Source: CAD feature listing. Evaluate the final solid. Frame: model axes, mm. Face numbers are marked on the shaded views. Give positions to 0.01 mm unless a question says otherwise; leave off trailing zeros. Loops run counter-clockwise (first coordinate to the right, second up) from the corner with the lowest first, then second, coordinate; pieces in that order, holes last. Notation, with made-up numbers: M 36,-1 L 89,-1 A30 cw 89,29 Z; hole C 59.25,-19 d7. An arc over 180 degrees is marked long. Answer in a Markdown table with one row per item.
```python
from build123d import *

# Parameters (mm, degrees)
SKETCH1_W           = 12
SKETCH1_H           = 30
BOSS_EXTRUDE1_DEPTH = 5
SKETCH2_R           = 2.25
CUT_EXTRUDE1_DEPTH  = 153.676695316
CHAMFER1_SIZE       = 2


with BuildPart() as part:
    # Sketch1 → Boss-Extrude1 (new body)
    with BuildSketch(Plane.XY):
        with Locations((127.56172091, 58.8)):
            Rectangle(SKETCH1_W, SKETCH1_H)
    extrude(amount=BOSS_EXTRUDE1_DEPTH)

    # Sketch2 → Cut-Extrude1 (cut, through all)
    with BuildSketch(Plane.XY.offset(5)):
        with Locations((127.56172091, 67.8)):
            Circle(SKETCH2_R)
        with Locations((127.56172091, 49.8)):
            Circle(SKETCH2_R)
    extrude(amount=-CUT_EXTRUDE1_DEPTH, mode=Mode.SUBTRACT)

    # Chamfer1
    # the kernel refuses this chamfer: 2 mm, written as the material it takes off along each edge
    with BuildSketch(Plane(origin=(133.56172091, 38.656634024, 5), x_dir=(0.027495876610582174, 0, -0.9996219169112968), z_dir=(0, 1, 0)), Plane(origin=(121.56172091, 78.943365976, 5), x_dir=(-0.02749587661058908, 0, -0.9996219169112968), z_dir=(0, -1, 0))) as chamfer1_piece_1:
        Polygon((CHAMFER1_SIZE * 0.999621916911, CHAMFER1_SIZE * 0.0274958766106), (-CHAMFER1_SIZE * 0.0274958766106, CHAMFER1_SIZE * 0.999621916911), (0, 0), align=None)
    extrude(amount=40.286731952, mode=Mode.SUBTRACT)
    with BuildSketch(Plane(origin=(127.56172091, 67.8, 5), x_dir=(1, 0, 0), z_dir=(0, -1, 0))) as chamfer1_piece_2:
        Polygon((2.25 + CHAMFER1_SIZE, 0), (2.25, -CHAMFER1_SIZE), (2.25, 0), align=None)
    revolve(axis=Axis((127.56172091, 67.8, 5), (0, 0, 1)), mode=Mode.SUBTRACT)
    with BuildSketch(Plane(origin=(138.705086886, 73.8, 5), x_dir=(0, 0.02749587661058908, -0.9996219169112968), z_dir=(-1, 0, 0))) as chamfer1_piece_3:
        Polygon((CHAMFER1_SIZE * 0.999621916911, CHAMFER1_SIZE * 0.0274958766106), (-CHAMFER1_SIZE * 0.0274958766106, CHAMFER1_SIZE * 0.999621916911), (0, 0), align=None)
    extrude(amount=22.286731952, mode=Mode.SUBTRACT)
    with BuildSketch(Plane(origin=(127.56172091, 49.8, 5), x_dir=(1, 0, 0), z_dir=(0, -1, 0))) as chamfer1_piece_4:
        Polygon((2.25 + CHAMFER1_SIZE, 0), (2.25, -CHAMFER1_SIZE), (2.25, 0), align=None)
    revolve(axis=Axis((127.56172091, 49.8, 5), (0, 0, 1)), mode=Mode.SUBTRACT)
    with BuildSketch(Plane(origin=(116.418354934, 43.8, 5), x_dir=(1.1837901526131779e-15, 0.9996219169112968, 0.02749587661058651), z_dir=(1, 0, 0))) as chamfer1_piece_5:
        Polygon((CHAMFER1_SIZE * 0.999621916911, -CHAMFER1_SIZE * 0.0274958766106), (-CHAMFER1_SIZE * 0.0274958766106, -CHAMFER1_SIZE * 0.999621916911), (0, 0), align=None)
    extrude(amount=22.286731952, mode=Mode.SUBTRACT)


solid = part.part
```
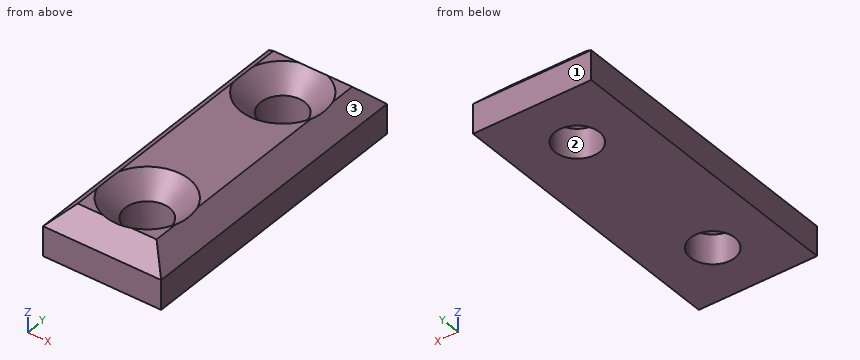
Q1. Contact query for flat-ended pins moving along their axis: pin 1 Ø6 at (x, y) = (127.56, 67.8) entering from +Z; pin 2 Ø3 at (y, z) = (63.5, 4) entering from +X; pin 3 Ø4 at (x, y) = (127.56, 49.8) entering from -Z. Output: stop coordinate, or through.
Values follow:
| item | result |
|---|---|
| pin 1 | z = 3.75 |
| pin 2 | x = 133.56 |
| pin 3 | through |
Q2. Section query C-C (y = 57.5). Output: boundary loops of the cut face in (x, z).
Values follow:
| item | result |
|---|---|
| outline | M 121.56,0 L 133.56,0 L 133.56,3 L 131.56,5 L 123.56,5 L 121.56,3 Z |
Q3. Section query A-A (y = 49.8). Output: boundary loops of the cut face in (x, z) (3 decimals).
Values follow:
| item | result |
|---|---|
| outline | M 121.562,0 L 125.312,0 L 125.312,3 L 123.437,4.875 L 121.562,3 Z; M 129.812,0 L 133.562,0 L 133.562,3 L 131.687,4.875 L 129.812,3 Z |
Q4. Ray query, probe 1 along Y at (x, z) = (128, 1.65); probe 2 along Y at (x, z) = (126, 2.8); probe 3 along X at (y, z) = (68, 3.85). Return the intervals inside material, ascending. Write a range as from..to.
Values follow:
| item | result |
|---|---|
| probe 1 | 43.8..47.59, 52.01..65.59, 70.01..73.8 |
| probe 2 | 43.8..48.18, 51.42..66.18, 69.42..73.8 |
| probe 3 | 122.41..124.47, 130.66..132.71 |
Q5. Section query D-D (x = 122.5). Output: boundary loops of the cut face in (y, z), plus the area to 3 significant figures.
Values follow:
| item | result |
|---|---|
| outline | M 43.8,0 L 73.8,0 L 73.8,3 L 72.86,3.94 L 44.74,3.94 L 43.8,3 Z |
| area | 117 mm^2 |
Q6. Section query B-B (z = 0.6). Output: boundary loops of the cut face in (x, y).
Values follow:
| item | result |
|---|---|
| outline | M 121.56,43.8 L 133.56,43.8 L 133.56,73.8 L 121.56,73.8 Z; hole C 127.56,49.8 d4.5; hole C 127.56,67.8 d4.5 |
Q7. Mould query, pull axis Y, two halves, no side actions, for the marked faces 1, 2 and 3. Classes: +Y half, -Y half, draft (parallel to the pull), parting line (faces both ways), or undercut.
Values follow:
| item | result |
|---|---|
| face 1 | +Y half |
| face 2 | undercut |
| face 3 | draft |
